CAD build for the part. Positions are in the model's coordinates, mm. A direction names the side the tool comes from. Coordinates: 2 decimals unless noted, no trailing zeros. Write each loop counter-clockwise with the first axis right and the second up, starting at its lowest first coordinate (ties: lowest second). Pieces come first, ordered by that corner, then holes. Notation, with made-up numbers: M 19,20 L 23,20 A16 ccw 23,42 Z; hole C 42,66 d10. An arc over 180 degrees is marked long. Put each result on its own line as item: value. Start each with the question number.
Autodesk Inventor part; units mm, degrees
ref_plane "YZ Plane" through (0, 0, 0) normal (1, 0, 0) x (0, 1, 0)
ref_plane "XZ Plane" through (0, 0, 0) normal (0, 1, 0) x (-1, 0, 0)
ref_plane "XY Plane" through (0, 0, 0) normal (0, 0, 1) x (1, 0, 0)
sketch "Sketch1" plane through (0, 0, 0) normal (0, 0, 1) x (1, 0, 0)
  circle A0 centre (0, 0) radius 6.35
  dimension "d0" = 12.7
extrude "Extrusion1" add sketch "Sketch1" against normal blind 50.8
sketch "Sketch2" plane through (0, 0, 0) normal (0, 0, 1) x (1, 0, 0)
  circle A0 centre (0, 0) radius 6.35
  circle A1 centre (0, 0) radius 19.05
  dimension "d3" = 38.1
extrude "Extrusion2" add sketch "Sketch2" against normal blind 6.35
sketch "Sketch4" plane through (0, 0, -6.35) normal (0, 0, -1) x (-1, 0, 0)
  circle A0 centre (0, 0) radius 19.05
  circle A1 centre (0, 0) radius 6.35 construction
  line L0 (0, 0) -> (0, 19.05) construction
  circle A2 centre (0, 0) radius 19.05 construction
  line L1 (-3.175, 18.7836) -> (-3.175, 15.6086)
  line L2 (-3.175, 15.6086) -> (0, 15.6086)
  line L3 (3.175, 18.7836) -> (3.175, 15.6086)
  line L4 (3.175, 15.6086) -> (0, 15.6086)
  arc A3 (3.175, 18.7836) -> (-3.175, 18.7836) centre (0, 0) ccw
  dimension "d6" = 3.175
  dimension "d7" = 3.175
extrude "Extrusion3" add sketch "Sketch4" along normal blind 25.4 contours L3 L4 L2 L1 A0 picked at (-1.4126, 16.7458)
properties part number "innerClutch" material "PET Plastic"
(1) Which spindle directions (+Z, -Z, +X, -X, +Y, -Y) get a long thin tool onto all of the face, cutting with end or side? Do faces 4 (the face through (0, 0, 0)), 5 (the face through (-3.175, 17, -19)), 6 (the face through (-1.38, -6.2, -28.26)), 7 (the face through (3.175, 17, -19)). Say none if no direction does.
(2) Slice it at C-C, the plane z = -8. Write the cut outline in (x, y) (3 decimals), then the cut area to 3 significant figures.
(3) Slice it at D-D, the plane z = -37.5. Write the cut outline in (x, y).
(4) Slice it at B-B, the plane y = 0. Write the cut outline in (x, z).
(5) Drop flat-ended pins along their axis: pin 1 (3 mm diameter, centred on y = 6, z = -36.5, fed in from -X); pin 2 (3 mm diameter, centred on x = 3, z = -24.5, fed in from -Y); pin 3 (3 mm diameter, centred on y = -4.5, z = -20, fed in from +X). Give the stop position or say it passes through.
(6) Slice it at A-A, the plane x = 0. Write the cut outline in (y, z), then the cut area to 3 significant figures.
(7) Drill centre lines: line 1 (Z direction, x = 11, y = 4); line 2 (X direction, y = -5, z = -33); line 3 (Y direction, x = 3, z = -4). Where is each one in solid material? Low to high. Write a range as [from, to].
(8) Two-plate mould, pull along Y, no slides. Class faces 1 (the face through (0, 17, -31.75)), 2 (the face through (1.4, 19, -7.6)), 3 (the face through (0, 15.609, -19)): +Y half, -Y half, draft (parallel to the pull), parting line (faces both ways), or undercut.
Result set:
1. face 4: +Z, +X, -X, +Y, -Y
1. face 5: -Z, -X, +Y
1. face 6: -Z
1. face 7: -Z, +X, +Y
2. outline: C 0,0 d12.7; M -3.175,15.609 L 3.175,15.609 L 3.175,18.784 A19.05 ccw -3.175,18.784 Z
2. area: 148 mm^2
3. outline: C 0,0 d12.7
4. outline: M -19.05,-6.35 L -6.35,-6.35 L -6.35,-50.8 L 6.35,-50.8 L 6.35,-6.35 L 19.05,-6.35 L 19.05,0 L -19.05,0 Z
5. pin 1: stops at x = -4.48
5. pin 2: stops at y = -6.17
5. pin 3: stops at x = 5.6
6. outline: M -19.05,-6.35 L -6.35,-6.35 L -6.35,-50.8 L 6.35,-50.8 L 6.35,-6.35 L 15.61,-6.35 L 15.61,-31.75 L 19.05,-31.75 L 19.05,0 L -19.05,0 Z
6. area: 894 mm^2
7. line 1: z = [-6.35, 0]
7. line 2: x = [-3.91, 3.91]
7. line 3: y = [-18.81, 18.81]
8. face 1: draft
8. face 2: parting line
8. face 3: undercut
